from build123d import *

# Parameters (mm, degrees)
SKETCH3_W          = 12.35
SKETCH3_H          = 7
CUT_EXTRUDE1_DEPTH = 10
CIRPATTERN1_COUNT  = 18


with BuildPart() as part:
    # Sketch1 → Revolve3 (revolve)
    with BuildSketch(Plane.XY):
        with BuildLine():
            Line((-24.170190138, 0.789195982), (-27.5, 16.23))
            Line((-27.5, 16.23), (-26.17011529, 16.23))
            Line((-26.17011529, 16.23), (-23.120650468, 2.089195982))
            ThreePointArc((-23.120650468, 2.089195982), (-22.771292475, 1.521924163), (-22.143122123, 1.3))
            Line((-22.143122123, 1.3), (-20.5, 1.3))
            Line((-20.5, 1.3), (-20.5, 0))
            Line((-20.5, 0), (-23.192661792, 0))
            ThreePointArc((-23.192661792, 0), (-23.820832144, 0.221924163), (-24.170190138, 0.789195982))
        make_face()
    revolve(axis=Axis((0, 0, 0), (0, 1, 0)))

    # Sketch3 → Cut-Extrude1 (cut)
    with BuildSketch(Plane(origin=(22.933479986, -4.945605665, 0), x_dir=(-0.210804018, -0.977528345, 0), z_dir=(0.977528345, -0.210804018, 0))):
        with Locations((-13.137395536, 0)):
            Rectangle(SKETCH3_W, SKETCH3_H)
    cut_extrude1 = extrude(amount=-CUT_EXTRUDE1_DEPTH, mode=Mode.SUBTRACT)

    # CirPattern1: Cut-Extrude1 ×18 about axis
    cirpattern1_axis = Axis((0, 0, 0), (0, 1, 0))
    for i in range(1, CIRPATTERN1_COUNT):
        add(cut_extrude1.rotate(cirpattern1_axis, i * 360 / CIRPATTERN1_COUNT), mode=Mode.SUBTRACT)


solid = part.part
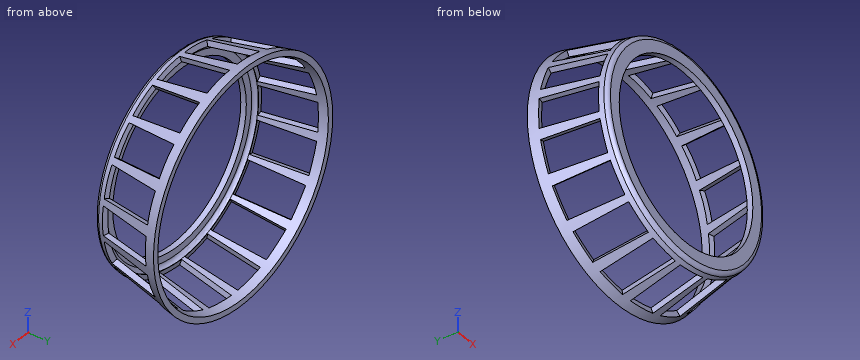
Can you work these out from the model? Positions are in its coordinate system, mm. Coordinates: 2 decimals unless noted, no trailing zeros. Loops run counter-clockwise (first coordinate to the right, second up) from the corner with the lowest first, then second, coordinate; pieces in that order, holes last. Notation, with made-up numbers: M 3,69.25 L 31,69.25 A24 ccw 31,106.25 Z; hole C 42,-9.5 d1. An arc over 180 degrees is marked long. Answer as CSV lines item,"result". Start each with the question number.
1. Suppose I cut it at A-A, the plane z = -2. Count the separate pieces of the cut face and the enclosed holes in it, plus the area to 3 significant figures.
2. For pin 1 Ø3 at (x, y) = (-12.5, 14) entering from -Z; pin 2 Ø4.5 at (x, y) = (25.5, 11) entering from -Z; pin 3 Ø3 at (x, y) = (-24, 8.5) entering from +Z; pin 4 Ø10 at (x, z) = (-6.5, 21) entering from +Y, each with a flat end and sliding along its axis, tell me the tip position at first contact or that it passes through.
3. Suppose I cut it at C-C, the plane y = 15.25. List the corners of the cut face in (x, z) for me, plus the area to 3 significant figures.
4. If I drill on probe 1 along Z at (x, y) = (0, 0.75); probe 2 along Z at (x, y) = (0, 0.3); probe 3 along Y at (x, z) = (21, 1), over which ranges is the centre line in solid material (lowest first)? Write a range as [from, to].
Output:
1,separate pieces,"4"
1,enclosed holes,"0"
1,area,"17.1 mm^2"
2,pin 1,"stops at z = -24.77"
2,pin 2,"stops at z = -12.57"
2,pin 3,"stops at z = 12.77"
2,pin 4,"stops at y = 16.23"
3,outline,"C 0,0 d54.58; hole C 0,0 d51.92"
3,area,"222 mm^2"
4,probe 1,"z = [-24.16, -20.5], [20.5, 24.16]"
4,probe 2,"z = [-23.91, -20.5], [20.5, 23.91]"
4,probe 3,"y = [0, 1.3]"
